Autodesk Inventor part; units mm, degrees
ref_plane "YZ Plane" through (0, 0, 0) normal (1, 0, 0) x (0, 1, 0)
ref_plane "XZ Plane" through (0, 0, 0) normal (0, 1, 0) x (-1, 0, 0)
ref_plane "XY Plane" through (0, 0, 0) normal (0, 0, 1) x (1, 0, 0)
sketch "Boceto1" plane through (0, 0, 0) normal (0, 1, 0) x (-1, 0, 0)
  circle A0 centre (0, 0) radius 35.165
  circle A1 centre (0, 0) radius 9.485
  circle A2 centre (0, 0) radius 14.45
  dimension "d0" = 70.33
  dimension "d23" = 18.97
  dimension "d24" = 28.9
extrude "Extrusión1" add sketch "Boceto1" along normal blind 26.85 contours A2
extrude "Extrusión2" add sketch "Boceto1" along normal blind 4.85 contours A0
thread "Rosca1"
sketch "Boceto2" plane through (0, 4.85, 0) normal (0, 1, 0) x (1, 0, 0)
  circle A0 centre (0, 0) radius 30.835
  dimension "d9" = 61.67
extrude "Extrusión3" cut sketch "Boceto2" against normal blind 1.67
sketch "Boceto3" plane through (0, 4.85, 0) normal (0, -1, 0) x (1, 0, 0)
  circle A0 centre (0, 0) radius 14.45
  circle A1 centre (0, 0) radius 9.485
extrude "Extrusión4" add sketch "Boceto3" along normal through all
sketch "Boceto4" plane through (0, 0, 0) normal (0, -1, 0) x (1, 0, 0)
  circle A0 centre (-20, 0) radius 3
  circle A1 centre (0, -20) radius 3
  circle A2 centre (20, 0) radius 3
  circle A3 centre (0, 20) radius 3
  point P0 (0, 0)
  dimension "d14" = 6
  dimension "d15" = 20
  dimension "d16" = 0
  dimension "d19" = 360
extrude "Extrusión5" cut sketch "Boceto4" against normal blind 26.85
properties part number "Flanche" material "PVC, no plastificado"
Geometry: final body of the model. Coordinates: model frame, mm. A direction names the side the tool comes from. Give positions to 0.01 mm unless a question says otherwise; leave off trailing zeros. Write each loop counter-clockwise with the first axis right and the second up, starting at its lowest first coordinate (ties: lowest second). Pieces come first, ordered by that corner, then holes. Notation, with made-up numbers: (-6, 39.25) -> (0, 39.25) arc R27 ccw to (0, 78.25) -> close; hole circle Ø2 at (19.25, 51). An arc over 180 degrees is marked (long way). Answer as a JSON object with one key per item and string values.
1. Cut plane A-A on x = 0. Output: boundary loops of the cut face in (y, z) (3 decimals), and give its area (3 significant figures).
Ans:
{"outline": "(0, -35.165) -> (4.85, -35.165) -> (4.85, -30.835) -> (3.18, -30.835) -> (3.18, -23) -> (0, -23) -> close; (0, -17) -> (3.18, -17) -> (3.18, -14.45) -> (26.85, -14.45) -> (26.85, -9.485) -> (0, -9.485) -> close; (0, 9.485) -> (26.85, 9.485) -> (26.85, 14.45) -> (3.18, 14.45) -> (3.18, 17) -> (0, 17) -> close; (0, 23) -> (3.18, 23) -> (3.18, 30.835) -> (4.85, 30.835) -> (4.85, 35.165) -> (0, 35.165) -> close", "area": "375 mm^2"}
2. Cut plane D-D on x = 20. Output: boundary loops of the cut face in (y, z), and give its area (3 significant figures).
Ans:
{"outline": "(0, -28.92) -> (4.85, -28.92) -> (4.85, -23.47) -> (3.18, -23.47) -> (3.18, -3) -> (0, -3) -> close; (0, 3) -> (3.18, 3) -> (3.18, 23.47) -> (4.85, 23.47) -> (4.85, 28.92) -> (0, 28.92) -> close", "area": "183 mm^2"}
3. Ray query, probe 1 along Z at (x, y) = (0, 2.4) (3 decimals); probe 2 along Y at (x, z) = (-9.5, -23.5); probe 3 along Z at (x, y) = (0, 21.5) (3 decimals). Return the intervals inside material, ascending. Write a range as from..to.
Ans:
{"probe 1": "z = -35.165..-23, -17..-9.485, 9.485..17, 23..35.165", "probe 2": "y = 0..3.18", "probe 3": "z = -14.45..-9.485, 9.485..14.45"}
4. Mould query, pull axis Z, two halves, no side actions, for faces 3 (the flat face through (0, 4.85, -31)), 4 (the cylindrical face through (-4.014, 4.027, -30.573)), 5 (the cylindrical face through (-33.54, 2.39, -10.56)). Classes: pulls with the +Z half, pulls with the -Z half, needs draft (parallel to the pull), parting line crosses it, or undercut.
Ans:
{"face 3": "needs draft", "face 4": "undercut", "face 5": "parting line crosses it"}
5. Cut plane C-C on y = 2.25. Output: boundary loops of the cut face in (x, z) (3 decimals), and give its area (3 significant figures).
Ans:
{"outline": "circle Ø70.33 at (0, 0); hole circle Ø6 at (-20, 0); hole circle Ø18.97 at (0, 0); hole circle Ø6 at (0, -20); hole circle Ø6 at (0, 20); hole circle Ø6 at (20, 0)", "area": "3,490 mm^2"}
6. Access query for faces 1 (the flat face through (13.3, 3.18, 6.4)), 2 (the cylindrical face through (-23, 2, 0)). Directions: +Z, -Z, +X, -X, +Y, -Y. A direction counts if a zero-diameter tool reaches every point of the face in a straight line with its end or side. Return the directions, or none.
Ans:
{"face 1": "+Y", "face 2": "+Y, -Y"}
7. Contact query for flat-ended pins moving along their axis: pin 1 (9.5 mm diameter, centred on x = 0, z = -20, fed in from -Y); pin 2 (6 mm diameter, centred on y = 19, z = 8.5, fed in from -X); pin 3 (4 mm diameter, centred on y = 9.5, z = -12.5, fed in from -X); pin 4 (1 mm diameter, centred on x = 12, z = -17, fed in from +Y). Output: stop coordinate, or through.
Ans:
{"pin 1": "stops at y = 0", "pin 2": "stops at x = -13.36", "pin 3": "stops at x = -9.93", "pin 4": "stops at y = 3.18"}
8. Cut plane B-B on z = 20. Output: boundary loops of the cut face in (x, y), and give its area (3 significant figures).
Ans:
{"outline": "(-28.92, 0) -> (-3, 0) -> (-3, 3.18) -> (-23.47, 3.18) -> (-23.47, 4.85) -> (-28.92, 4.85) -> close; (3, 0) -> (28.92, 0) -> (28.92, 4.85) -> (23.47, 4.85) -> (23.47, 3.18) -> (3, 3.18) -> close", "area": "183 mm^2"}
